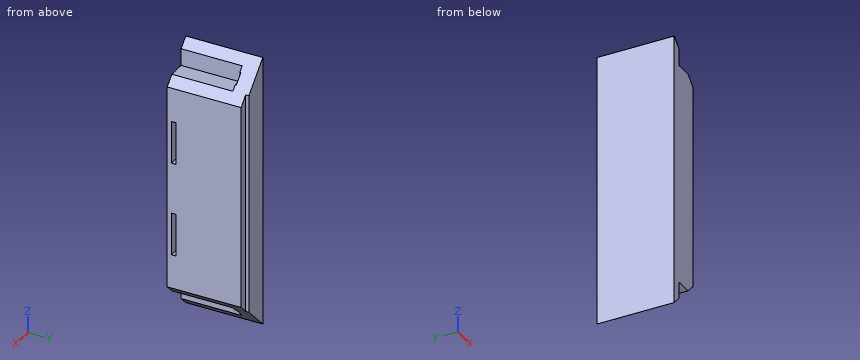
Autodesk Inventor part; units mm, degrees
ref_plane "YZ Plane" through (0, 0, 0) normal (1, 0, 0) x (0, 1, 0)
ref_plane "XZ Plane" through (0, 0, 0) normal (0, 1, 0) x (-1, 0, 0)
ref_plane "XY Plane" through (0, 0, 0) normal (0, 0, 1) x (1, 0, 0)
sketch "Sketch1" plane through (0, 0, 0) normal (0, 0, 1) x (1, 0, 0)
  line L0 (0, 0) -> (0, 228.6)
  line L1 (0, 228.6) -> (76.2, 228.6)
  line L2 (76.2, 228.6) -> (76.2, 219.2528)
  line L3 (76.2, 219.2528) -> (101.6, 219.2528)
  line L4 (101.6, 219.2528) -> (101.6, 0)
  line L5 (101.6, 0) -> (0, 0)
  dimension "d0" = 228.6
  dimension "d1" = 76.2
  dimension "d2" = 9.3472
  dimension "d3" = 25.4
extrude "Extrusion1" add sketch "Sketch1" along normal blind 812.8
sketch "Sketch6" plane through (0, 0, 0) normal (0, -1, 0) x (1, 0, 0)
  line L0 (101.6, 0) -> (101.6, 812.8)
  line L1 (0, 812.8) -> (101.6, 711.2)
  line L2 (76.2038, 736.5962) -> (25.4038, 736.5962)
  line L3 (25.4038, 736.5962) -> (25.4038, 787.3962)
  line L4 (25.4038, 787.3962) -> (76.2, 736.6)
  point P0 (0, 0)
  point P1 (101.6, 101.6)
  dimension "d31" = 35.9156
  dimension "d32" = 50.8
  dimension "d33" = 50.8
extrude "Extrusion4" cut sketch "Sketch6" against normal blind 181.1528
sketch "Sketch7" plane through (25.4038, 0, 736.5962) normal (0, -1, 0) x (1, 0, 0)
  line L0 (76.1962, -634.9962) -> (50.7962, -660.3962)
  line L1 (50.7962, -660.3962) -> (-0.0038, -660.3962)
  line L2 (76.1962, -634.9962) -> (-25.4038, -736.5962)
  line L3 (76.1962, -736.5962) -> (76.1962, 76.2038)
  line L4 (-0.0038, -660.3962) -> (-0.0038, -711.1962)
  line L5 (-0.0038, -711.1962) -> (50.7962, -660.3962)
  point P0 (76.1962, -25.3962)
  dimension "d39" = 50.8
  dimension "d41" = 90
  dimension "d42" = 50.8
extrude "Extrusion5" cut sketch "Sketch7" against normal blind 181.1528
chamfer "Chamfer5" distance 101.6 angle 45 1 edges at (101.6, 109.6264, 812.8)
chamfer "Chamfer6" distance 101.6 angle 45 1 edges at (101.6, 109.6264, 0)
sketch "Sketch8" plane through (25.4038, 181.1528, 736.5962) normal (0, -1, 0) x (1, 0, 0)
  line L0 (-25.4038, -736.5962) -> (50.7962, -660.3962)
  line L1 (50.7962, -660.3962) -> (38.0981, -673.0942)
  line L2 (38.0981, -673.0942) -> (12.6981, -673.0942)
  line L3 (12.6981, -673.0942) -> (12.6981, -698.4942)
  dimension "d54" = 17.9578
  dimension "d55" = 25.4
  dimension "d56" = 25.4
extrude "Extrusion6" cut sketch "Sketch8" against normal blind 3.175
sketch "Sketch9" plane through (0, 181.1528, 0) normal (0, -1, 0) x (1, 0, 0)
  line L0 (76.2, 736.6) -> (63.5019, 749.2981)
  line L1 (38.1019, 749.2981) -> (63.5019, 749.2981)
  line L2 (38.1019, 749.2981) -> (38.1019, 774.6981)
  line L3 (38.1019, 774.6981) -> (63.5019, 749.2981)
  line L4 (25.4038, 787.3962) -> (76.2038, 736.5962)
  point P0 (0, 0)
extrude "Extrusion8" cut sketch "Sketch9" against normal blind 3.175
sketch "Sketch10" plane through (101.6, 0, 711.2) normal (1, 0, 0) x (0, 0, -1)
  line L0 (609.6, 219.2528) -> (0, 219.2528)
  line L1 (609.6, 219.2528) -> (609.6, 0)
  line L2 (609.6, 219.2528) -> (609.6, 0)
  line L3 (609.6, 0) -> (609.6, 12.7)
  line L4 (508, 12.7) -> (381, 12.7)
  line L5 (228.6, 12.7) -> (101.6, 12.7)
  line L6 (508, 12.7) -> (508, 25.4)
  line L7 (508, 25.4) -> (381, 25.4)
  line L8 (381, 25.4) -> (381, 12.7)
  line L9 (228.6, 12.7) -> (228.6, 25.4)
  line L10 (228.6, 25.4) -> (101.6, 25.4)
  line L11 (101.6, 25.4) -> (101.6, 12.7)
  point P0 (711.2, 0)
  dimension "d70" = 12.7
  dimension "d71" = 101.6
  dimension "d72" = 127
  dimension "d73" = 152.4
  dimension "d74" = 127
  dimension "d75" = 12.7
  dimension "d76" = 12.7
  dimension "d77" = 193.8528
extrude "Extrusion9" cut sketch "Sketch10" against normal blind 50.8 contours L5 L11 L10 L9
sketch "Sketch11" plane through (101.6, 0, 711.2) normal (1, 0, 0) x (0, 0, -1)
  line L0 (609.6, 219.2528) -> (0, 219.2528)
  line L1 (609.6, 219.2528) -> (609.6, 0)
  line L2 (609.6, 219.2528) -> (609.6, 0)
  line L3 (609.6, 0) -> (609.6, 12.7)
  line L4 (508, 12.7) -> (381, 12.7)
  line L5 (228.6, 12.7) -> (101.6, 12.7)
  line L6 (508, 12.7) -> (508, 25.4)
  line L7 (508, 25.4) -> (381, 25.4)
  line L8 (381, 25.4) -> (381, 12.7)
  line L9 (228.6, 12.7) -> (228.6, 25.4)
  line L10 (228.6, 25.4) -> (101.6, 25.4)
  line L11 (101.6, 25.4) -> (101.6, 12.7)
  point P0 (711.2, 0)
  point P1 (711.2, 0)
  dimension "d80" = 12.7
  dimension "d81" = 101.6
  dimension "d82" = 127
  dimension "d83" = 152.4
  dimension "d84" = 127
  dimension "d85" = 12.7
  dimension "d86" = 12.7
  dimension "d87" = 193.8528
extrude "Extrusion10" cut sketch "Sketch11" against normal blind 50.8 contours L4 L8 L7 L6
properties part number "SideWidth" material "Wood (Birch)"
Could you check a few things on this model? Use its own coordinates, in mm. Coordinates: 2 decimals unless noted, no trailing zeros. Loops run counter-clockwise (first coordinate to the right, second up) from the corner with the lowest first, then second, coordinate; pieces in that order, holes last.
1. Imagine slicing it at D-D (x = 18). Please give me the cut outline in (y, z).
2. Imagine slicing it at C-C (x = 89.5). Please give me the cut outline in (y, z).
3. For P1, Ø20.5, axis at x = 49.5, z = 45, coming from the -Y side; P2, Ø12, axis at x = 47.5, z = 513.5, coming from the -Y side; P3, Ø1.5, axis at x = 29, y = 70.5, coming from the -Z side; P4, Ø6.5, axis at x = 80.5, y = 18, coming from the -Z side, each with a flat end and sliding along its axis, tell me the tip position at first contact or that it passes through.
4. Imagine slicing it at A-A (y = 111). Please give me the cut outline in (x, z), and give its area (3 significant figures).
5. I need wall thicknesses on L1, parallel to Y at x = 60.5, z = 483; L2, parallel to Z at x = 74.5, y = 20.5; L3, parallel to Z at x = 54, y = 86. Which ranges of each line are inside material? Lowest first, please.
6. Imagine slicing it at B-B (z = 322). Please give me the cut outline in (x, y).
Computed values:
1. outline: (0, 18) - (228.6, 18) - (228.6, 794.8) - (0, 794.8) - close
2. outline: (0, 89.5) - (219.25, 89.5) - (219.25, 723.3) - (0, 723.3) - close; hole (12.7, 203.2) - (25.4, 203.2) - (25.4, 330.2) - (12.7, 330.2) - close; hole (12.7, 482.6) - (25.4, 482.6) - (25.4, 609.6) - (12.7, 609.6) - close
3. P1: stops at y = 184.33
3. P2: stops at y = 0
3. P3: stops at z = 76.2
3. P4: stops at z = 77.25
4. outline: (0, 0) - (25.4, 25.4) - (25.4, 76.2) - (76.2, 76.2) - (101.6, 101.6) - (101.6, 711.2) - (76.2, 736.6) - (25.4, 736.6) - (25.4, 787.4) - (0, 812.8) - close
4. area: 69,700 mm2
5. L1: y = 0 to 12.7, 25.4 to 228.6
5. L2: z = 76.2 to 203.2, 330.2 to 482.6, 609.6 to 736.6
5. L3: z = 76.2 to 736.6
6. outline: (0, 0) - (101.6, 0) - (101.6, 12.7) - (50.8, 12.7) - (50.8, 25.4) - (101.6, 25.4) - (101.6, 219.25) - (76.2, 219.25) - (76.2, 228.6) - (0, 228.6) - close
